```python
from build123d import *

# Parameters (mm, degrees)
SKETCH_1_R      = 41
SKETCH_1_R_2    = 33.05
SKETCH_1_R_3    = 1.5
EXTRUDE_1_DEPTH = 3.1


with BuildPart() as part:
    # 草图1 → 凸台-拉伸1 (new body)
    with BuildSketch(Plane.XY):
        with Locations(Location((0, 0, 0), (0, 0, 180))):
            Circle(SKETCH_1_R)
        with Locations(Location((0, 0, 0), (0, 0, 180))):
            Circle(SKETCH_1_R_2, mode=Mode.SUBTRACT)
        with Locations(Location((0, 37, 0), (0, 0, 180))):
            Circle(SKETCH_1_R_3, mode=Mode.SUBTRACT)
        with Locations(Location((18.5, 32.04293994, 0), (0, 0, 180))):
            Circle(SKETCH_1_R_3, mode=Mode.SUBTRACT)
        with Locations(Location((32.04293994, 18.5, 0), (0, 0, 180))):
            Circle(SKETCH_1_R_3, mode=Mode.SUBTRACT)
        with Locations(Location((37, 0, 0), (0, 0, 180))):
            Circle(SKETCH_1_R_3, mode=Mode.SUBTRACT)
        with Locations(Location((32.04293994, -18.5, 0), (0, 0, 180))):
            Circle(SKETCH_1_R_3, mode=Mode.SUBTRACT)
        with Locations(Location((18.5, -32.04293994, 0), (0, 0, 180))):
            Circle(SKETCH_1_R_3, mode=Mode.SUBTRACT)
        with Locations(Location((0, -37, 0), (0, 0, 180))):
            Circle(SKETCH_1_R_3, mode=Mode.SUBTRACT)
        with Locations(Location((-18.5, -32.04293994, 0), (0, 0, 180))):
            Circle(SKETCH_1_R_3, mode=Mode.SUBTRACT)
        with Locations(Location((-32.04293994, -18.5, 0), (0, 0, 180))):
            Circle(SKETCH_1_R_3, mode=Mode.SUBTRACT)
        with Locations(Location((-37, 0, 0), (0, 0, 180))):
            Circle(SKETCH_1_R_3, mode=Mode.SUBTRACT)
        with Locations(Location((-32.04293994, 18.5, 0), (0, 0, 180))):
            Circle(SKETCH_1_R_3, mode=Mode.SUBTRACT)
        with Locations(Location((-18.5, 32.04293994, 0), (0, 0, 180))):
            Circle(SKETCH_1_R_3, mode=Mode.SUBTRACT)
    extrude(amount=EXTRUDE_1_DEPTH)


solid = part.part
```
Input: part model. Units: mm. Frame: model coordinates. Round coordinates to 2 decimals unless told otherwise and drop trailing zeros. Loops run counter-clockwise (first coordinate to the right, second up) from the corner with the lowest first, then second, coordinate; pieces in that order, holes last. Notation, with made-up numbers: (6, 61) -> (36, 61) arc R21 cw to (36, 81) -> close; hole circle Ø3 at (-0.5, 14). An arc over 180 degrees is marked (long way). One line per item, written item: value.
(1) Section C-C (z = 1.9). Give the number of separate pieces and of enclosed holes in the cut face, plus the area to 3 significant figures.
Geometry check:
separate pieces: 1
enclosed holes: 13
area: 1,760 mm2
(2) Section D-D (y = -4). Return the cut outline in (x, z).
Geometry check:
outline: (-40.8, 0) -> (-32.81, 0) -> (-32.81, 3.1) -> (-40.8, 3.1) -> close; (32.81, 0) -> (40.8, 0) -> (40.8, 3.1) -> (32.81, 3.1) -> close
(3) Mould query, pull axis Y, two halves, no side actions, for faces 1 (the face through (-37.874, 15.703, 1.528)), 2 (the face through (0.2, 33.2, 3.1)), 3 (the face through (-17, -32, 2)). Classes: pulls with the +Y half, pulls with the -Y half, needs draft (parallel to the pull), parting line crosses it, or undercut.
Geometry check:
face 1: parting line crosses it
face 2: needs draft
face 3: undercut
(4) Section B-B (y = 18.5). Return the cut outline in (x, z), plus the area to 3 significant figures.
Geometry check:
outline: (-36.59, 0) -> (-33.54, 0) -> (-33.54, 3.1) -> (-36.59, 3.1) -> close; (-30.54, 0) -> (-27.39, 0) -> (-27.39, 3.1) -> (-30.54, 3.1) -> close; (27.39, 0) -> (30.54, 0) -> (30.54, 3.1) -> (27.39, 3.1) -> close; (33.54, 0) -> (36.59, 0) -> (36.59, 3.1) -> (33.54, 3.1) -> close
area: 38.5 mm2
(5) Material intervals for line 1 (Y direction, x = 1, z = 2.25); line 2 (Y direction, x = -18.5, z = 0.7), sorted ascending. Write a range as [from, to].
Geometry check:
line 1: [-40.99, -38.12], [-35.88, -33.03], [33.03, 35.88], [38.12, 40.99]
line 2: [-36.59, -33.54], [-30.54, -27.39], [27.39, 30.54], [33.54, 36.59]
(6) Pin query (flat end, axial travel): pin 1 (3.5 mm diameter, centred on x = 18.5, y = 32.04, fed in from +Z); pin 2 (1 mm diameter, centred on x = -18.5, z = 0.5, fed in from -Y); pin 3 (1.5 mm diameter, centred on y = 14.5, z = 1.5, fed in from -X). Return the tip coordinate at first contact, or that it passes through.
Geometry check:
pin 1: z = 3.1
pin 2: y = -36.84
pin 3: x = -38.63
(7) Section A-A (x = 0). Return the cut outline in (y, z).
Geometry check:
outline: (-41, 0) -> (-38.5, 0) -> (-38.5, 3.1) -> (-41, 3.1) -> close; (-35.5, 0) -> (-33.05, 0) -> (-33.05, 3.1) -> (-35.5, 3.1) -> close; (33.05, 0) -> (35.5, 0) -> (35.5, 3.1) -> (33.05, 3.1) -> close; (38.5, 0) -> (41, 0) -> (41, 3.1) -> (38.5, 3.1) -> close
